Verification items for the finished model (mm, model axes). A direction names the side the tool comes from. Round coordinates to 2 decimals unless told otherwise and drop trailing zeros. Order: outer loops, then holes, each group sorted by start corner. A loop starts at its lowest first (then second) coordinate and runs counter-clockwise, first axis right, second up. Notation, with made-up numbers: (9, 7.25) -> (24, 7.25) arc R25 ccw to (24, 21.25) -> close; hole circle Ø11 at (78.5, 61.25). An arc over 180 degrees is marked (long way). Put each result on its own line as item: value.
from build123d import *

# Parameters (mm, degrees)
BOSS_EXTRUDE1_DEPTH             = 76.2
BOSS_EXTRUDE1_DEPTH_BACK        = 76.2
CUT_EXTRUDE1_DEPTH              = 136.619651209
CUT_EXTRUDE1_DEPTH_BACK         = 136.619651209
FILLET1_R                       = 3.81
SHELL1_START                    = -44.45
SHELL1_DEPTH                    = 88.773
SHELL1_START_2                  = -73.025
SHELL1_2_DEPTH                  = 130.048
SKETCH14_R                      = 1.984375
CUT_EXTRUDE8_DEPTH              = 156.372005628
BOSS_EXTRUDE4_REACH             = 137.201
SKETCH15_R                      = 1.5875
BOSS_EXTRUDE4_DIRECTION_2_REACH = 137.201


# Read off the part's stored shape, not the designer's step: Shell1
with BuildPart() as part:
    # Sketch1 → Boss-Extrude1 (new, two sides: drawn at the far end of the back side and taken through both)
    with BuildSketch(Plane.XY.offset(-BOSS_EXTRUDE1_DEPTH_BACK)):
        with BuildLine():
            Line((-6.335258536, -105.245804705), (-12.685258536, -3.645804705))
            ThreePointArc((-12.685258536, -3.645804705), (0.014741464, 8.866413132), (12.714741464, -3.645804705))
            Line((12.714741464, -3.645804705), (6.364741464, -105.245804705))
            ThreePointArc((6.364741464, -105.245804705), (0.014741464, -111.465623147), (-6.335258536, -105.245804705))
        make_face()
    extrude(amount=BOSS_EXTRUDE1_DEPTH + BOSS_EXTRUDE1_DEPTH_BACK)

    # Sketch4 → Cut-Extrude1 (cut, two sides: drawn at the far end of the back side and taken through both)
    with BuildSketch(Plane(origin=(0, 0, 0), x_dir=(0, 0, -1), z_dir=(1, 0, 0)).offset(-CUT_EXTRUDE1_DEPTH_BACK)):
        Polygon((-47.498, -73.524605007), (-47.498, -51.299605007), (47.625, -51.299605007), (47.625, -73.524605007), (76.2, -73.524605007), (76.2, 8.866413132), (-76.2, 8.866413132), (-76.2, -28.682279346), (-76.2, -111.465623147), (-60.198, -111.465623147), (-60.198, -73.524605007), align=None)
    extrude(amount=CUT_EXTRUDE1_DEPTH + CUT_EXTRUDE1_DEPTH_BACK, mode=Mode.SUBTRACT)

    # Fillet1
    fillet1_edges = [part.edges().sort_by_distance(p)[0] for p in [
        (8.347316445, -73.524605007, 53.848),
        (9.736378945, -51.299605007, -0.0635),
        (-9.706896017, -51.299605007, -0.0635),
        (-8.317833517, -73.524605007, 53.848),
        (-8.317833517, -73.524605007, -61.9125),
        (8.347316445, -73.524605007, -61.9125),
    ]]
    fillet(fillet1_edges, radius=FILLET1_R)

    # Shell1 outline → Shell1 (cut)
    with BuildSketch(Plane.XY.offset(SHELL1_START)):
        with BuildLine():
            ThreePointArc((-3.161602106, -105.125185529), (0.014741465, -108.290623147), (3.191085035, -105.125185529))
            Line((3.191085035, -105.125185529), (6.314583179, -55.149215219))
            ThreePointArc((6.314583179, -55.149215219), (6.143625088, -54.674822007), (5.680819792, -54.474605007))
            Line((5.680819792, -54.474605007), (-5.651336863, -54.474605007))
            ThreePointArc((-5.651336863, -54.474605007), (-6.114142159, -54.674822006), (-6.285100251, -55.149215219))
            Line((-6.285100251, -55.149215219), (-3.161602106, -105.125185529))
        make_face()
    extrude(amount=SHELL1_DEPTH, mode=Mode.SUBTRACT)

    # Shell1 2 outline → Shell1 2 (cut)
    with BuildSketch(Plane.XY.offset(SHELL1_START_2)):
        with BuildLine():
            Line((-4.896037751, -77.374215219), (-3.161602106, -105.125185529))
            ThreePointArc((-3.161602106, -105.125185529), (0.014741465, -108.290623147), (3.191085035, -105.125185529))
            Line((3.191085035, -105.125185529), (4.925520679, -77.374215219))
            ThreePointArc((4.925520679, -77.374215219), (4.754562588, -76.899822007), (4.291757292, -76.699605007))
            Line((4.291757292, -76.699605007), (-4.262274363, -76.699605007))
            ThreePointArc((-4.262274363, -76.699605007), (-4.725079659, -76.899822006), (-4.896037751, -77.374215219))
        make_face()
    extrude(amount=SHELL1_2_DEPTH, mode=Mode.SUBTRACT)

    # Sketch14 → Cut-Extrude8 (cut, through all)
    with BuildSketch(Plane(origin=(0, 0, -47.625), x_dir=(-1, 0, 0), z_dir=(0, 0, -1))):
        with Locations((-0.014741464, -61.459605007)):
            Circle(SKETCH14_R)
    extrude(amount=-CUT_EXTRUDE8_DEPTH, mode=Mode.SUBTRACT)

    # Boss-Extrude4: up to this plane
    boss_extrude4_end = Plane(origin=(3.195924528, -105.047753647, -76.2), z_dir=(0.9980525784828886, -0.062378286155180485, 0))
    # Sketch15 → Boss-Extrude4 (add, up to the surface)
    with BuildSketch(Plane(origin=(3.191103822, -0.502900096, 0), x_dir=(0, 0, -1), z_dir=(1, 0, 0)), mode=Mode.PRIVATE) as boss_extrude4_sk1:
        with Locations(Location((-9.398, -66.274366182, 0), (0, 0, 270))):
            Circle(SKETCH15_R)
    boss_extrude4_tool1 = split(extrude(boss_extrude4_sk1.sketch, amount=BOSS_EXTRUDE4_REACH, mode=Mode.PRIVATE), bisect_by=boss_extrude4_end, keep=Keep.BOTH, mode=Mode.PRIVATE)
    add(boss_extrude4_tool1.solids().sort_by_distance((3.191104, -66.777266, 9.398))[0])
    # Sketch15 → Boss-Extrude4 (add, up to the surface)
    with BuildSketch(Plane(origin=(3.191103822, -0.502900096, 0), x_dir=(0, 0, -1), z_dir=(1, 0, 0)), mode=Mode.PRIVATE) as boss_extrude4_sk2:
        with Locations(Location((26.868345804, -77.595887652, 0), (0, 0, 270))):
            Circle(SKETCH15_R)
    boss_extrude4_tool2 = split(extrude(boss_extrude4_sk2.sketch, amount=BOSS_EXTRUDE4_REACH, mode=Mode.PRIVATE), bisect_by=boss_extrude4_end, keep=Keep.BOTH, mode=Mode.PRIVATE)
    add(boss_extrude4_tool2.solids().sort_by_distance((3.191104, -78.098788, -26.868346))[0])
    # Sketch15 → Boss-Extrude4 (add, up to the surface)
    with BuildSketch(Plane(origin=(3.191103822, -0.502900096, 0), x_dir=(0, 0, -1), z_dir=(1, 0, 0)), mode=Mode.PRIVATE) as boss_extrude4_sk3:
        with Locations(Location((-22.098, -96.55076585, 0), (0, 0, 270))):
            Circle(SKETCH15_R)
    boss_extrude4_tool3 = split(extrude(boss_extrude4_sk3.sketch, amount=BOSS_EXTRUDE4_REACH, mode=Mode.PRIVATE), bisect_by=boss_extrude4_end, keep=Keep.BOTH, mode=Mode.PRIVATE)
    add(boss_extrude4_tool3.solids().sort_by_distance((3.191104, -97.053666, 22.098))[0])
    # Sketch15 → Boss-Extrude4 (add, up to the surface)
    with BuildSketch(Plane(origin=(3.191103822, -0.502900096, 0), x_dir=(0, 0, -1), z_dir=(1, 0, 0)), mode=Mode.PRIVATE) as boss_extrude4_sk4:
        with Locations(Location((16.002, -96.55076585, 0), (0, 0, 270))):
            Circle(SKETCH15_R)
    boss_extrude4_tool4 = split(extrude(boss_extrude4_sk4.sketch, amount=BOSS_EXTRUDE4_REACH, mode=Mode.PRIVATE), bisect_by=boss_extrude4_end, keep=Keep.BOTH, mode=Mode.PRIVATE)
    add(boss_extrude4_tool4.solids().sort_by_distance((3.191104, -97.053666, -16.002))[0])
    # Sketch15 → Boss-Extrude4 (add, up to the surface)
    with BuildSketch(Plane(origin=(3.191103822, -0.502900096, 0), x_dir=(0, 0, -1), z_dir=(1, 0, 0)), mode=Mode.PRIVATE) as boss_extrude4_sk5:
        with Locations(Location((54.102, -96.55076585, 0), (0, 0, 270))):
            Circle(SKETCH15_R)
    boss_extrude4_tool5 = split(extrude(boss_extrude4_sk5.sketch, amount=BOSS_EXTRUDE4_REACH, mode=Mode.PRIVATE), bisect_by=boss_extrude4_end, keep=Keep.BOTH, mode=Mode.PRIVATE)
    add(boss_extrude4_tool5.solids().sort_by_distance((3.191104, -97.053666, -54.102))[0])

    # Boss-Extrude4 direction 2: up to this plane
    boss_extrude4_direction_2_end = Plane(origin=(-3.166441599, -105.047753647, -76.2), z_dir=(-0.9980525784828886, -0.0623782861551806, 0))
    # Sketch15 → Boss-Extrude4 direction 2 (add, up to the surface)
    with BuildSketch(Plane(origin=(3.191103822, -0.502900096, 0), x_dir=(0, 0, -1), z_dir=(1, 0, 0)), mode=Mode.PRIVATE) as boss_extrude4_direction_2_sk1:
        with Locations(Location((-9.398, -66.274366182, 0), (0, 0, 270))):
            Circle(SKETCH15_R)
    boss_extrude4_direction_2_tool1 = split(extrude(boss_extrude4_direction_2_sk1.sketch, amount=-BOSS_EXTRUDE4_DIRECTION_2_REACH, mode=Mode.PRIVATE), bisect_by=boss_extrude4_direction_2_end, keep=Keep.BOTH, mode=Mode.PRIVATE)
    add(boss_extrude4_direction_2_tool1.solids().sort_by_distance((3.191104, -66.777266, 9.398))[0])
    # Sketch15 → Boss-Extrude4 direction 2 (add, up to the surface)
    with BuildSketch(Plane(origin=(3.191103822, -0.502900096, 0), x_dir=(0, 0, -1), z_dir=(1, 0, 0)), mode=Mode.PRIVATE) as boss_extrude4_direction_2_sk2:
        with Locations(Location((26.868345804, -77.595887652, 0), (0, 0, 270))):
            Circle(SKETCH15_R)
    boss_extrude4_direction_2_tool2 = split(extrude(boss_extrude4_direction_2_sk2.sketch, amount=-BOSS_EXTRUDE4_DIRECTION_2_REACH, mode=Mode.PRIVATE), bisect_by=boss_extrude4_direction_2_end, keep=Keep.BOTH, mode=Mode.PRIVATE)
    add(boss_extrude4_direction_2_tool2.solids().sort_by_distance((3.191104, -78.098788, -26.868346))[0])
    # Sketch15 → Boss-Extrude4 direction 2 (add, up to the surface)
    with BuildSketch(Plane(origin=(3.191103822, -0.502900096, 0), x_dir=(0, 0, -1), z_dir=(1, 0, 0)), mode=Mode.PRIVATE) as boss_extrude4_direction_2_sk3:
        with Locations(Location((-22.098, -96.55076585, 0), (0, 0, 270))):
            Circle(SKETCH15_R)
    boss_extrude4_direction_2_tool3 = split(extrude(boss_extrude4_direction_2_sk3.sketch, amount=-BOSS_EXTRUDE4_DIRECTION_2_REACH, mode=Mode.PRIVATE), bisect_by=boss_extrude4_direction_2_end, keep=Keep.BOTH, mode=Mode.PRIVATE)
    add(boss_extrude4_direction_2_tool3.solids().sort_by_distance((3.191104, -97.053666, 22.098))[0])
    # Sketch15 → Boss-Extrude4 direction 2 (add, up to the surface)
    with BuildSketch(Plane(origin=(3.191103822, -0.502900096, 0), x_dir=(0, 0, -1), z_dir=(1, 0, 0)), mode=Mode.PRIVATE) as boss_extrude4_direction_2_sk4:
        with Locations(Location((16.002, -96.55076585, 0), (0, 0, 270))):
            Circle(SKETCH15_R)
    boss_extrude4_direction_2_tool4 = split(extrude(boss_extrude4_direction_2_sk4.sketch, amount=-BOSS_EXTRUDE4_DIRECTION_2_REACH, mode=Mode.PRIVATE), bisect_by=boss_extrude4_direction_2_end, keep=Keep.BOTH, mode=Mode.PRIVATE)
    add(boss_extrude4_direction_2_tool4.solids().sort_by_distance((3.191104, -97.053666, -16.002))[0])
    # Sketch15 → Boss-Extrude4 direction 2 (add, up to the surface)
    with BuildSketch(Plane(origin=(3.191103822, -0.502900096, 0), x_dir=(0, 0, -1), z_dir=(1, 0, 0)), mode=Mode.PRIVATE) as boss_extrude4_direction_2_sk5:
        with Locations(Location((54.102, -96.55076585, 0), (0, 0, 270))):
            Circle(SKETCH15_R)
    boss_extrude4_direction_2_tool5 = split(extrude(boss_extrude4_direction_2_sk5.sketch, amount=-BOSS_EXTRUDE4_DIRECTION_2_REACH, mode=Mode.PRIVATE), bisect_by=boss_extrude4_direction_2_end, keep=Keep.BOTH, mode=Mode.PRIVATE)
    add(boss_extrude4_direction_2_tool5.solids().sort_by_distance((3.191104, -97.053666, -54.102))[0])


solid = part.part
Item 1: Section check A-A on z = -3.5. Record the boundary of the cut face in (x, y) (3 decimals), then the cut area to 3 significant figures.
Check sheet entries:
outline: (-9.454, -55.347) -> (-6.335, -105.246) arc R6.351 ccw to (6.365, -105.246) -> (9.483, -55.347) arc R3.81 ccw to (5.681, -51.3) -> (-5.651, -51.3) arc R3.81 ccw to start; hole (-6.285, -55.149) -> (-3.162, -105.125) arc R3.176 ccw to (3.191, -105.125) -> (6.315, -55.149) arc R0.635 ccw to (5.681, -54.475) -> (-5.651, -54.475) arc R0.635 ccw to start
area: 424 mm^2
Item 2: Gauge pin test, flat ends, axial feed: pin 1 Ø8 at (y, z) = (-72, 16) entering from +X; pin 2 Ø8 at (y, z) = (-94.5, -4.5) entering from -X; pin 3 Ø4.5 at (x, y) = (0.01, -61.46) entering from -Z (3 decimals); pin 4 Ø10 at (y, z) = (-66, -59) entering from +X. Record the tip position at first contact, or that the pin passes through.
Check sheet entries:
pin 1: stops at x = 8.69
pin 2: stops at x = -7.26
pin 3: stops at z = -47.625
pin 4: passes through
Item 3: Material ranges on L1, parallel to Z at x = 0.75, y = -104.5 (3 decimals); L2, parallel to Z at x = -4.75, y = -79 (3 decimals); L3, parallel to Z at x = 6.25, y = -54 (3 decimals), recorded low to high. Write a range as [from, to].
Check sheet entries:
L1: z = [-76.2, -73.025], [57.023, 60.198]
L2: z = [-76.2, -73.025], [-28.175, -25.561], [57.023, 60.198]
L3: z = [-47.625, 47.498]
Item 4: Section check C-C on y = -83.5. Record the boundary of the cut face in (x, z) (3 decimals).
Check sheet entries:
outline: (-7.694, -76.2) -> (7.724, -76.2) -> (7.724, 60.198) -> (-7.694, 60.198) -> close; hole (-4.513, -73.025) -> (4.543, -73.025) -> (4.543, 57.023) -> (-4.513, 57.023) -> close
Item 5: Section check D-D on y = -102. Record the boundary of the cut face in (x, z) (3 decimals).
Check sheet entries:
outline: (-6.538, -76.2) -> (6.568, -76.2) -> (6.568, 60.198) -> (-6.538, 60.198) -> close; hole (-3.357, -73.025) -> (3.386, -73.025) -> (3.386, 57.023) -> (-3.357, 57.023) -> close
Item 6: Section check B-B on y = -72. Record the boundary of the cut face in (x, z) (3 decimals), then the cut area to 3 significant figures.
Check sheet entries:
outline: (-8.413, -47.625) -> (8.443, -47.625) -> (8.443, 47.498) -> (-8.413, 47.498) -> close; hole (-5.232, -44.45) -> (5.261, -44.45) -> (5.261, 44.323) -> (-5.232, 44.323) -> close
area: 672 mm^2
Item 7: Release check for a two-part mould opening along X. For faces 1 (the flat face through (0, -65, 47.498)), 2 (the flat face through (0, -76.7, -59)), 3 (the cylindrical face through (0.153, -111.464, -8.956)), 4 (the flat face through (7.946, -79.947, -8.956)) record: +X half, -X half, draft (parallel to the pull), parting line (faces both ways), or undercut.
Check sheet entries:
face 1: draft
face 2: undercut
face 3: parting line
face 4: +X half
Item 8: Tool access check on faces 5 (the flat face through (0, -92, 57.023)), 6 (the flat face through (0, -73.525, -62)), 7 (the flat face through (0, -92, -76.2)). Record the directions out of +Z, -Z, +X, -X, +Y, -Y that give a thin tool (end or side, any length) a straight path to the whole face; none if there is none.
Check sheet entries:
face 5: none
face 6: -Z, +X, -X, +Y
face 7: -Z, +X, -X, +Y, -Y
